from build123d import *

# Parameters (mm, degrees)
SKETCH1_R           = 69.723
SKETCH1_R_2         = 66.548
BOSS_EXTRUDE1_DEPTH = 76.2
SKETCH2_R           = 22.479
SKETCH2_R_2         = 19.304
BOSS_EXTRUDE2_DEPTH = 6.35
BOSS_EXTRUDE3_START = -6.35
BOSS_EXTRUDE3_DEPTH = 6.35
CIRPATTERN1_COUNT   = 3
FILLET4_R           = 7.62
FILLET6_R           = 1.016


with BuildPart() as part:
    # Sketch1 → Boss-Extrude1 (new body)
    with BuildSketch(Plane(origin=(0, 0, 0), x_dir=(1, 0, 0), z_dir=(0, 1, 0))):
        with Locations(Location((0, 0, 0), (0, 0, 90))):
            Circle(SKETCH1_R)
        with Locations(Location((0, 0, 0), (0, 0, 90))):
            Circle(SKETCH1_R_2, mode=Mode.SUBTRACT)
    extrude(amount=BOSS_EXTRUDE1_DEPTH)



with BuildPart() as body_2:
    # Sketch2 → Boss-Extrude2 (new body)
    with BuildSketch(Plane(origin=(0, 76.2, 0), x_dir=(1, 0, 0), z_dir=(0, 1, 0))):
        with Locations(Location((0, 0, 0), (0, 0, 270))):
            Circle(SKETCH2_R)
        with Locations(Location((0, 0, 0), (0, 0, 270))):
            Circle(SKETCH2_R_2, mode=Mode.SUBTRACT)
    extrude(amount=-BOSS_EXTRUDE2_DEPTH)


with BuildPart() as part_1:
    add(part.part)

    add(body_2.part)  # Boss-Extrude3 merges body 2
    # Sketch3 → Boss-Extrude3 (add)
    with BuildSketch(Plane(origin=(0, 76.2, 0), x_dir=(1, 0, 0), z_dir=(0, 1, 0)).offset(BOSS_EXTRUDE3_START)):
        with BuildLine():
            Line((-1.5875, 22.422874141), (-1.5875, 66.52906243))
            ThreePointArc((-1.5875, 66.52906243), (0, 66.548), (1.5875, 66.52906243))
            Line((1.5875, 66.52906243), (1.5875, 22.422874141))
            ThreePointArc((1.5875, 22.422874141), (0, 22.479), (-1.5875, 22.422874141))
        make_face()
    boss_extrude3 = extrude(amount=BOSS_EXTRUDE3_DEPTH)

    # CirPattern1: Boss-Extrude3 ×3 about axis
    cirpattern1_axis = Axis((0, 0, 0), (0, 1, 0))
    for i in range(1, CIRPATTERN1_COUNT):
        add(boss_extrude3.rotate(cirpattern1_axis, i * 360 / CIRPATTERN1_COUNT))

    # Sketch5 → Revolve2 (revolve)
    with BuildSketch(Plane.XY, mode=Mode.PRIVATE) as revolve2_sk:
        Polygon((66.52906243, 76.2), (107.346075645, 124.843822138), (110.540013215, 124.843822138), (69.723, 76.2), align=None)
    revolve(revolve2_sk.sketch.rotate(Axis((0, 76.2, 0), (0, -1, 0)), 90), axis=Axis((0, 76.2, 0), (0, -1, 0)))

    # Fillet4
    # the kernel refuses this fillet: 7.62 mm, written as the material it adds along each edge
    with BuildSketch(Plane(origin=(1.5875, 69.85, -22.422874141), x_dir=(0.9818555419021507, 0, 0.18963041643163103), z_dir=(0, 1, 0)), Plane(origin=(-20.212528632, 69.85, 9.836621742), x_dir=(-0.3267030129910606, 0, -0.9451270503496146), z_dir=(0, 1, 0)), Plane(origin=(18.625028632, 69.85, 12.586252399), x_dir=(-0.6551525289110903, 0, 0.7554966339179832), z_dir=(0, 1, 0))) as fillet4_piece_1:
        with BuildLine():
            CenterArc((6.299731081, 7.565105602), FILLET4_R, 190.931216516, 72.187250076)
            Line((-1.182008148, 6.120121829), (0, 0))
            ThreePointArc((0, 0), (2.693363288, 0.161938473), (5.386726576, 0))
        make_face()
    extrude(amount=6.35)
    with BuildSketch(Plane(origin=(-1.5875, 69.85, -22.422874141), x_dir=(0, 0, -1), z_dir=(0, 1, 0)), Plane(origin=(-18.625028632, 69.85, 12.586252399), x_dir=(-0.8660254037844387, 0, 0.49999999999999983), z_dir=(0, 1, 0))) as fillet4_piece_2:
        with BuildLine():
            CenterArc((6.233220232, 7.62), FILLET4_R, 197.812749924, 72.187250076)
            ThreePointArc((-1.021487204, 5.288987342), (-0.351743415, 2.675202131), (0, 0))
            Line((0, 0), (6.233220232, 0))
        make_face()
    extrude(amount=6.35)
    with BuildSketch(Plane(origin=(-1.5875, 69.85, -66.52906243), x_dir=(-0.9959189542007358, 0, 0.09025207290534944), z_dir=(0, 1, 0)), Plane(origin=(-56.822108154, 69.85, 34.639346543), x_dir=(0.5761200649806046, 0, 0.8173650779955944), z_dir=(0, 1, 0))) as fillet4_piece_3:
        with BuildLine():
            CenterArc((8.340236793, 7.60314841), FILLET4_R, 174.821891179, 98.989299345)
            Line((0.751334362, 8.290869205), (0, 0))
            ThreePointArc((0, 0), (4.423364453, -0.147170556), (8.846728906, 0))
        make_face()
    extrude(amount=6.35)
    with BuildSketch(Plane(origin=(1.5875, 69.85, -66.52906243), x_dir=(0, 0, 1), z_dir=(0, 1, 0))) as fillet4_piece_4:
        with BuildLine():
            CenterArc((8.324843272, 7.62), FILLET4_R, 171.010700655, 98.989299345)
            ThreePointArc((0.798435622, 8.810625), (0.252647865, 4.418594948), (0, 0))
            Line((0, 0), (8.324843272, 0))
        make_face()
    extrude(amount=6.35)
    with BuildSketch(Plane(origin=(-58.409608154, 69.85, 31.889715886), x_dir=(-0.41979888922013026, 0, -0.9076171509009427), z_dir=(0, 1, 0)), Plane(origin=(56.822108154, 69.85, 34.639346543), x_dir=(-0.5761200649806054, 0, 0.8173650779955935), z_dir=(0, 1, 0))) as fillet4_piece_5:
        with BuildLine():
            CenterArc((8.340236793, -7.60314841), FILLET4_R, 86.188809476, 98.989299345)
            Line((0.751334362, -8.290869205), (0, 0))
            ThreePointArc((0, 0), (4.423364453, 0.147170556), (8.846728906, 0))
        make_face()
    extrude(amount=6.35)
    with BuildSketch(Plane(origin=(20.212528632, 69.85, 9.836621742), x_dir=(0.32670301299106214, 0, -0.9451270503496141), z_dir=(0, 1, 0))) as fillet4_piece_6:
        with BuildLine():
            CenterArc((6.299731081, -7.565105602), FILLET4_R, 96.881533408, 72.187250076)
            Line((-1.182008148, -6.120121829), (0, 0))
            ThreePointArc((0, 0), (2.693363288, -0.161938473), (5.386726576, 0))
        make_face()
    extrude(amount=6.35)
    with BuildSketch(Plane(origin=(58.409608154, 69.85, 31.889715886), x_dir=(-0.8660254037844388, 0, -0.49999999999999967), z_dir=(0, 1, 0))) as fillet4_piece_7:
        with BuildLine():
            CenterArc((8.324843272, -7.62), FILLET4_R, 90, 98.989299345)
            ThreePointArc((0.798435622, -8.810625), (0.252647865, -4.418594948), (0, 0))
            Line((0, 0), (8.324843272, 0))
        make_face()
    extrude(amount=6.35)

    # Fillet6
    fillet6_edges = [part_1.edges().sort_by_distance(p)[0] for p in [
        (0, 124.843822138, -110.540013215),
        (0, 124.843822138, -107.346075645),
    ]]
    fillet(fillet6_edges, radius=FILLET6_R)


solid = part_1.part
Can you work these out from the model? Positions are in its coordinate system, mm. A direction names the side the tool comes from. Round coordinates to 2 decimals unless told otherwise and drop trailing zeros. Loops run counter-clockwise (first coordinate to the right, second up) from the corner with the lowest first, then second, coordinate; pieces in that order, holes last. Notation, with made-up numbers: (49.5, 41.5) - (75.5, 41.5) arc R33 ccw to (75.5, 70.5) - close; hole circle Ø7 at (85, 45.5). An arc over 180 degrees is marked (long way). Use CSV: the item, a comma, the result in double quotes. Start each with the question number.
1) If we section it at B-B on z = 0: Count the separate pieces of the cut face and the enclosed holes in it, plus the area to 3 significant figures.
2) If we section it at D-D on y = 93.5: Write out the boundary of the cut face in (x, z), plus the area to 3 significant figures.
3) For faces 3 (the flat face through (-1.588, 73, -43)), 4 (the flat face through (17, 69.85, 10)), which set-ups out of +Z, -Z, +X, -X, +Y, -Y let a thin tool reach every point of the face, with its end or its side?
4) We'd pull the mould along Z, two halves only. Please class faces 1 (the conical face through (69.93, 78.48, -15.53)), 2 (the cylindrical face through (-57.64, 72.98, 28.28)): released by +Z, released by -Z, zero draft, split by the parting line, or undercut.
5) For pin 1 Ø7.5 at (x, z) = (-23, 56) entering from -Y; pin 2 Ø7 at (y, z) = (72.5, -50) entering from +X; pin 3 Ø1.5 at (y, z) = (105, 52) entering from +X (3 decimals); pin 4 Ø10 at (x, y) = (10, 74) entering from -Z, each with a flat end and sliding along its axis, tell me the tip position at first contact or that it passes through.
6) Please list where these lines run through material, in increasing order: probe 1 along X at (y, z) = (75, 0); probe 2 along X at (y, z) = (35, 0); probe 3 along Z at (x, y) = (-8.5, 51). Write a range as [from, to].
7) If we section it at A-A on y = 30.5: Write out the boundary of the cut face in (x, z), plus the area to 3 significant figures.
Geometry results:
1,separate pieces,"4"
1,enclosed holes,"0"
1,area,"833 mm2"
2,outline,"circle Ø168.48 at (0, 0); hole circle Ø162.09 at (0, 0)"
2,area,"1,660 mm2"
3,face 3,"+Y, -Y"
3,face 4,"-Y"
4,face 1,"split by the parting line"
4,face 2,"undercut"
5,pin 1,"passes through"
5,pin 2,"stops at x = 51.95"
5,pin 3,"stops at x = 79.075"
5,pin 4,"stops at z = -71.43"
6,probe 1,"x = [-69.72, -66.55], [-22.48, -19.3], [19.3, 22.48], [66.55, 69.72]"
6,probe 2,"x = [-69.72, -66.55], [66.55, 69.72]"
6,probe 3,"z = [-69.2, -66], [66, 69.2]"
7,outline,"circle Ø139.45 at (0, 0); hole circle Ø133.1 at (0, 0)"
7,area,"1,360 mm2"
